Source: three-view drawing plus pictorial views. Frame: mm from the lowest corner of the part. A direction names the side the tool comes from. Give positions to 0.01 mm unless a question says otherwise; leave off trailing zeros. Write each loop counter-clockwise with the first axis right and the second up, starting at its lowest first coordinate (ties: lowest second). Pieces come first, ordered by that corner, then holes. Notation, with made-up numbers: (25.5, 23) -> (77.5, 23) arc R31 ccw to (77.5, 61) -> close; hole circle Ø5 at (48.5, 89.25). An arc over 180 degrees is marked (long way). Answer in a Markdown table with one row per item. Add a question column.
Item 1: Draft query along X for the marked faces 4, 5 and 6. Return one class per face: +X half, -X half, draft (parallel to the pull), parting line (faces both ways), or undercut.
Item 2: Access query for the marked faces 1, 2 and 3. Directions: +Z, -Z, +X, -X, +Y, -Y. A direction counts if a zero-diameter tool reaches every point of the face in a straight line with its end or side. Return the directions, or none.
Item 3: Section query D-D on x = 25. Output: boundary loops of the cut face in (y, z).
Item 4: First-contact query: P1, Ø1.5, axis at y = 27.5, z = 0.5, coming from the +X side; P2, Ø1.5, axis at x = 12, z = 3.5, coming from the -Y side; P3, Ø0.6, axis at y = 34.5, z = 2.5, coming from the +X side; P4, Ø3, axis at y = 20, z = 3.5, coming from the +X side. Flat tips, straight axial feed; report the tip coordinate or a pass-through.
Item 5: Material intervals for probe 1 along X at (y, z) = (10, 1.7); probe 2 along X at (y, z) = (24, 2.2) (1 decimal); probe 3 along Y at (x, z) = (32, 1.25), sorted ascending. Write a range as from..to.
Item 6: Section query C-C on z = 3.25. Output: boundary loops of the cut face in (x, y).
Item 7: Section query B-B on y = 9. Output: boundary loops of the cut face in (x, z) (1 decimal).
Item 8: Section query A-A on x = 5.5. Output: boundary loops of the cut face in (y, z), plus the area to 3 significant figures.
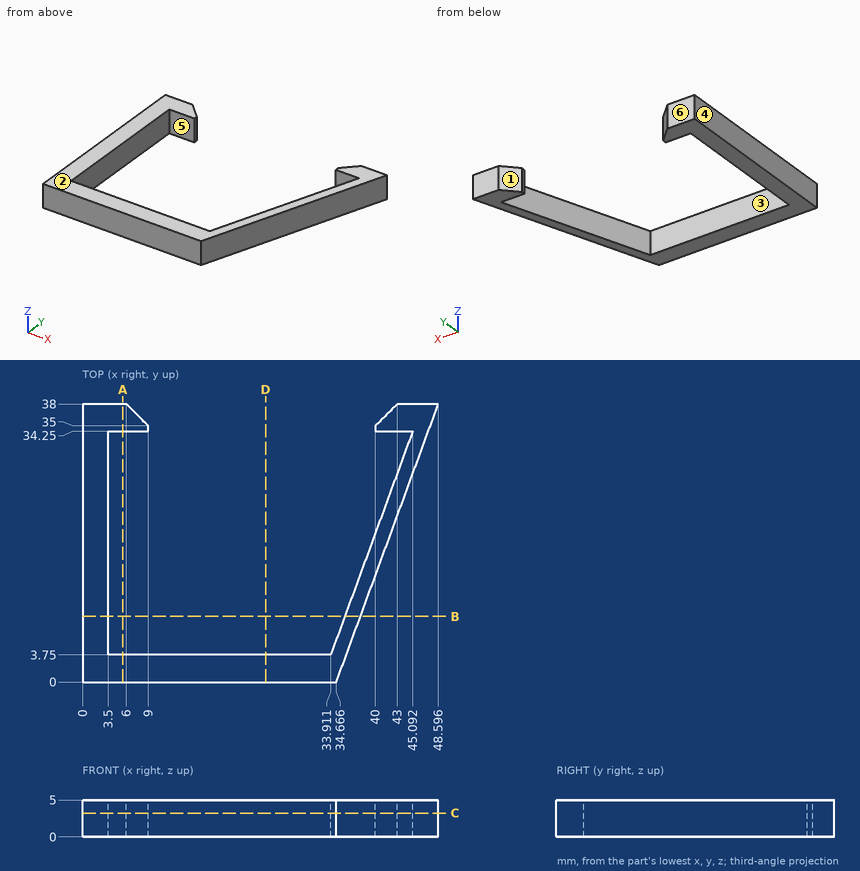
Findings below:
| question | item | result |
|---|---|---|
| 1 | face 4 | -X half |
| 1 | face 5 | undercut |
| 1 | face 6 | draft |
| 2 | face 1 | +Z, -Z, +Y |
| 2 | face 2 | +Z, +X, -X, +Y, -Y |
| 2 | face 3 | +Z, -Z |
| 3 | outline | (0, 0) -> (3.75, 0) -> (3.75, 5) -> (0, 5) -> close |
| 4 | P1 | stops at x = 45.02 |
| 4 | P2 | stops at y = 0 |
| 4 | P3 | stops at x = 47.42 |
| 4 | P4 | stops at x = 42.55 |
| 5 | probe 1 | x = 0..3.5, 36.2..38.33 |
| 5 | probe 2 | x = 0..3.5, 41.3..43.5 |
| 5 | probe 3 | y = 0..3.75 |
| 6 | outline | (0, 0) -> (34.67, 0) -> (48.6, 38) -> (43, 38) -> (40, 35) -> (40, 34.25) -> (45.09, 34.25) -> (33.91, 3.75) -> (3.5, 3.75) -> (3.5, 34.25) -> (9, 34.25) -> (9, 35) -> (6, 38) -> (0, 38) -> close |
| 7 | outline | (0, 0) -> (3.5, 0) -> (3.5, 5) -> (0, 5) -> close; (35.8, 0) -> (38, 0) -> (38, 5) -> (35.8, 5) -> close |
| 8 | outline | (0, 0) -> (3.75, 0) -> (3.75, 5) -> (0, 5) -> close; (34.25, 0) -> (38, 0) -> (38, 5) -> (34.25, 5) -> close |
| 8 | area | 37.5 mm^2 |
